Build history of the part. All positions in model axes, mm. Face numbers are marked on the shaded views. A direction names the side the tool comes from. Round coordinates to 2 decimals unless told otherwise and drop trailing zeros. Order: outer loops, then holes, each group sorted by start corner. A loop starts at its lowest first (then second) coordinate and runs counter-clockwise, first axis right, second up. Notation, with made-up numbers: (69.5, 33) -> (118.5, 33) arc R26 cw to (118.5, 68) -> close; hole circle Ø1 at (1.25, 61.25). An arc over 180 degrees is marked (long way). Write item = value, one per line.
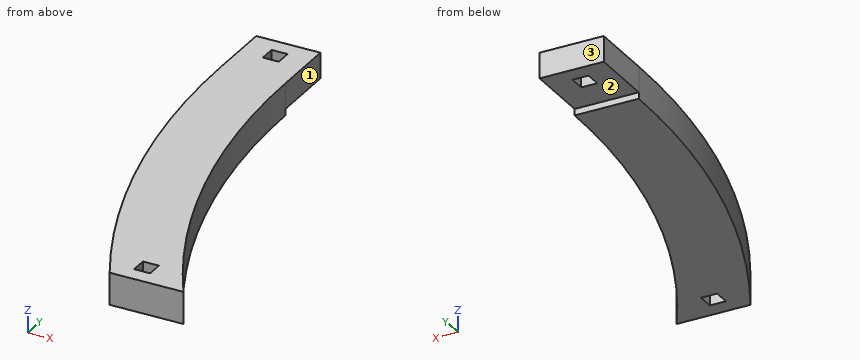
Autodesk Inventor part; units mm, degrees
ref_plane "YZ Plane" through (0, 0, 0) normal (1, 0, 0) x (0, 1, 0)
ref_plane "XZ Plane" through (0, 0, 0) normal (0, 1, 0) x (-1, 0, 0)
ref_plane "XY Plane" through (0, 0, 0) normal (0, 0, 1) x (1, 0, 0)
sketch "Sketch1" plane through (0, 0, 0) normal (0, 0, 1) x (1, 0, 0)
  circle A0 centre (0, 0) radius 292.1
  line L0 (-292.1, 0) -> (-266.7, 0)
  line L1 (-292.1, 0) -> (-317.5, 0)
  circle A1 centre (0, 0) radius 317.5
  line L2 (-317.5, 0) -> (-317.5, -150.4188)
  line L3 (-317.5, -150.4188) -> (-250.3929, -150.4188)
  circle A2 centre (0, 0) radius 317.5
  dimension "d0" = 584.2
  dimension "d1" = 25.4
  dimension "d2" = 25.4
  dimension "d3" = 150.4188
extrude "Extrusion1" add sketch "Sketch1" along normal blind 12.7 contours A0 L3 A1 L1 | A1 L3 L2 picked at (-273.7775, -123.6883)
sketch "Sketch2" plane through (0, 0, 12.7) normal (0, 0, 1) x (1, 0, 0)
  line L0 (-317.5, 0) -> (-317.5, -150.4188)
  line L1 (-317.5, -150.4188) -> (-250.3929, -150.4188)
  arc A0 (-292.1, 0) -> (-250.3929, -150.4188) centre (0, 0) ccw
  circle A1 centre (0, 0) radius 292.1
  circle A2 centre (0, 0) radius 317.5
  line L2 (-317.5, 0) -> (-317.5, -150.4188)
  line L3 (-317.5, -150.4188) -> (-279.6076, -150.4188)
extrude "Extrusion2" cut sketch "Sketch2" against normal blind 25.4 contours A2 L1 L0
sketch "Sketch3" plane through (0, 0, 12.7) normal (0, 0, 1) x (1, 0, 0)
  arc A0 (-317.5, 0) -> (-279.6076, -150.4188) centre (0, 0) ccw
  arc A1 (-292.1, 0) -> (-250.3929, -150.4188) centre (0, 0) ccw
  line L0 (-279.6076, -150.4188) -> (-304.8, -150.4188)
  line L1 (-284.5263, -140.8938) -> (-284.5263, -150.4188)
  line L2 (-284.5263, -140.8938) -> (-255.8737, -140.8938)
  line L3 (-270.2, -137.7188) -> (-267.025, -137.7188)
  line L4 (-267.025, -137.7188) -> (-267.025, -144.0688)
  line L5 (-267.025, -144.0688) -> (-273.375, -144.0688)
  line L6 (-273.375, -144.0688) -> (-273.375, -137.7188)
  line L7 (-273.375, -137.7188) -> (-270.2, -137.7188)
  dimension "d14" = 9.525
  dimension "d16" = 3.175
  dimension "d17" = 6.35
  dimension "d18" = 6.35
  dimension "d19" = 3.175
  dimension "d20" = 4.9186
  dimension "d21" = 11.1513
extrude "Extrusion3" cut sketch "Sketch3" against normal blind 25.4
sketch "Sketch4" plane through (0, 0, 12.7) normal (0, 0, 1) x (1, 0, 0)
  arc A0 (-317.5, 0) -> (-279.6076, -150.4188) centre (0, 0) ccw
  arc A1 (-292.1, 0) -> (-250.3929, -150.4188) centre (0, 0) ccw
  line L0 (-292.1, 0) -> (-317.5, 0)
  line L1 (-317.5, 0) -> (-317.5, 25.4)
  line L2 (-317.5, 25.4) -> (-292.1, 25.4)
  line L3 (-292.1, 25.4) -> (-292.1, 0)
  line L4 (-317.5, 0) -> (-292.1, 0)
  dimension "d24" = 25.4
extrude "Extrusion4" add sketch "Sketch4" against normal blind 10.16
sketch "Sketch5" plane through (0, 0, 12.7) normal (0, 0, 1) x (1, 0, 0)
  line L0 (-292.1, 0) -> (-292.1, 25.4)
  line L1 (-292.1, 25.4) -> (-317.5, 25.4)
  line L2 (-317.5, 25.4) -> (-317.5, 0)
  line L3 (-304.8, 25.4) -> (-304.8, 19.05)
  line L4 (-304.8, 19.05) -> (-301.625, 19.05)
  line L5 (-301.625, 19.05) -> (-301.625, 12.7)
  line L6 (-301.625, 12.7) -> (-307.975, 12.7)
  line L7 (-307.975, 12.7) -> (-307.975, 19.05)
  line L8 (-307.975, 19.05) -> (-304.8, 19.05)
  dimension "d27" = 6.35
  dimension "d28" = 3.175
  dimension "d29" = 6.35
  dimension "d30" = 6.35
extrude "Extrusion5" cut sketch "Sketch5" against normal blind 10.16
properties part number "HopperFrontSupport_v1"
Q1. Probe probe 1 along X at (y, z) = (16.5, 9.25) (3 decimals); probe 2 along Z at (x, y) = (-308, 6.5); probe 3 along X at (y, z) = (-62, 2.5). List the from-to ranges inside material, lowest first.
Check values:
probe_1 = -317.5 to -307.975, -301.625 to -292.1
probe_2 = 2.54 to 12.7
probe_3 = -311.39 to -285.44
Q2. Which spindle directions (+Z, -Z, +X, -X, +Y, -Y) get a long thin tool onto all of the face, cutting with end or side? Do the marked faces 1, 2 and 3. Say none if no direction does.
Check values:
face_1 = +Z, -Z, +X, +Y
face_2 = -Z, +X, -X, +Y
face_3 = +Z, -Z, +X, -X, +Y
Q3. Cut at C-C, the plane y = 4. List the corners of the cut face in (x, z), and give its area (3 significant figures).
Check values:
outline = (-317.5, 2.54) -> (-292.1, 2.54) -> (-292.1, 12.7) -> (-317.5, 12.7) -> close
area = 258 mm²
Q4. Flat gauge pins, fed straight in: pin 1 (12.5 mm diameter, centred on x = -305.5, y = 10, fed in from -Z); pin 2 (5 mm diameter, centred on y = -141.5, z = 3, fed in from -X); pin 3 (2 mm diameter, centred on y = -104, z = 1.5, fed in from +X); pin 4 (4 mm diameter, centred on x = -291, z = 9, fed in from +Y). Where does each tip first touch, or does it go through?
Check values:
pin_1 = 2.54
pin_2 = -285.46
pin_3 = -272.58
pin_4 = 25.4
Q5. Cut at B-B, the plane x = -306. List the corners of the cut face in (y, z), and give its area (3 significant figures).
Check values:
outline = (-84.68, 0) -> (0, 0) -> (0, 2.54) -> (12.7, 2.54) -> (12.7, 12.7) -> (-84.68, 12.7) -> close; (19.05, 2.54) -> (25.4, 2.54) -> (25.4, 12.7) -> (19.05, 12.7) -> close
area = 1,270 mm²
Q6. Cut at D-D, the plane y = -119. List the corners of the cut face in (x, z), and give its area (3 significant figures).
Check values:
outline = (-294.36, 0) -> (-266.76, 0) -> (-266.76, 12.7) -> (-294.36, 12.7) -> close
area = 350 mm²
Q7. Cut at A-A, the plane z = 8.5. List the corners of the cut face in (x, y) (3 decimals).
Check values:
outline = (-317.5, 0) arc R317.5 ccw to (-279.608, -150.419) -> (-250.393, -150.419) arc R292.1 cw to (-292.1, 0) -> (-292.1, 25.4) -> (-317.5, 25.4) -> close; hole (-307.975, 12.7) -> (-301.625, 12.7) -> (-301.625, 19.05) -> (-307.975, 19.05) -> close; hole (-273.375, -144.069) -> (-267.025, -144.069) -> (-267.025, -137.719) -> (-273.375, -137.719) -> close
